Source: CAD feature listing. Evaluate the final solid. Frame: model axes, mm. A direction names the side the tool comes from. Coordinates: 2 decimals unless noted, no trailing zeros. Write each loop counter-clockwise with the first axis right and the second up, starting at its lowest first coordinate (ties: lowest second). Pieces come first, ordered by that corner, then holes. Notation, with made-up numbers: M -29,-36.75 L -11,-36.75 A6 ccw -11,-29.75 Z; hole C 73,-40 d11. An arc over 180 degrees is marked long. One line per item, written item: value. Start each with the question number.
Item 1: Ray query, L1, parallel to X at y = 0, z = 101.75; L2, parallel to Y at x = 0, z = 94.5; L3, parallel to Z at x = 5, y = 5.5. Return the intervals inside material, ascending. Write a range as from..to.
Item 2: Pin query (flat end, axial travel): P1, Ø5, axis at y = -1, z = 36, coming from the -X side (3 decimals); P2, Ø10.5, axis at y = -2.5, z = 17.5, coming from the -X side; P3, Ø5, axis at x = 20, z = 85, coming from the -Y side. Return the tip coordinate at first contact, or that it passes through.
Item 3: Cut plane A-A, the plane z = 18.5. Output: boundary loops of the cut face in (x, y), then the cut area to 3 significant figures.
Item 4: Set-up query: faces 4 (the flat face through (-7.89, -13.92, 15.91)), 5 (the flat face through (-6, -16, 91)), 6 (the conical face through (-14.35, 8.33, 22.16)), 7 (the flat face through (-16, 0, 100)). Return all of +Z, -Z, +X, -X, +Y, -Y with unobstructed straight access to the full face (end or side cutting, diameter ignored); none if empty.
Item 5: Cut plane B-B, the plane z = 81. Output: boundary loops of the cut face in (x, y).
Item 6: Mould query, pull axis Y, two halves, no side actions, for faces 1 (the conical face through (-11.986, -1.574, 38.389)), 2 (the flat face through (-17, -9, 45)), 3 (the flat face through (-7.89, 13.92, 99.62)). Classes: released by +Y, released by -Y, zero draft, split by the parting line, or undercut.
```python
from build123d import *

# Parameters (mm, degrees)
SKETCH_2_R          = 33
SKETCH_2_W          = 44
SKETCH_2_H          = 22
CUT_EXTRUDE_1_DEPTH = 6.5
SKETCH_3_R          = 33
SKETCH_3_W          = 22
SKETCH_3_H          = 44
CUT_EXTRUDE_2_DEPTH = 6.5
SKETCH_5_R          = 32
CUT_EXTRUDE_3_DEPTH = 17
SKETCH_7_R          = 32
CUT_EXTRUDE_4_DEPTH = 13


with BuildPart() as part:
    # 草图1 → 旋转1 (revolve)
    with BuildSketch(Plane(origin=(0, 0, 0), x_dir=(0, 0, -1), z_dir=(1, 0, 0))):
        Polygon((-83, 0), (-83, 10.188), (-107.188, 10.188), (-108, 11), (-108, 16), (-106.57093764, 18.475208614), (-91.6, 18.475208614), (-91, 19.075208614), (-91, 24.5), (-89, 26.5), (-52, 26.5), (-45, 22.933321854), (-45, 10.5), (-38.5, 10.5), (-38.5, 11.8), (-38.3, 12), (-32.2, 12), (-32, 11.8), (-32, 11), (-0.92, 11), (0, 10.08), (0, 0), align=None)
    revolve(axis=Axis((0, 0, 0), (0, 0, 1)))

    # 草图2 → 切除-拉伸1 (cut)
    with BuildSketch(Plane(origin=(0, 0, 32), x_dir=(-1, 0, 0), z_dir=(0, 0, -1))):
        Circle(SKETCH_2_R)
        Rectangle(SKETCH_2_W, SKETCH_2_H, mode=Mode.SUBTRACT)
    extrude(amount=-CUT_EXTRUDE_1_DEPTH, mode=Mode.SUBTRACT)

    # 草图3 → 切除-拉伸2 (cut)
    with BuildSketch(Plane(origin=(0, 0, 32), x_dir=(-1, 0, 0), z_dir=(0, 0, -1))):
        Circle(SKETCH_3_R)
        Rectangle(SKETCH_3_W, SKETCH_3_H, mode=Mode.SUBTRACT)
    extrude(amount=-CUT_EXTRUDE_2_DEPTH, mode=Mode.SUBTRACT)

    # 草图4 → 旋转2 (revolve)
    with BuildSketch(Plane(origin=(0, 0, 0), x_dir=(0, 0, -1), z_dir=(1, 0, 0))):
        with BuildLine():
            Line((-45, 19), (-45, 10.5))
            Line((-45, 10.5), (-38.5, 10.5))
            Line((-38.5, 10.5), (-38.5, 11.8))
            Line((-38.5, 11.8), (-36.726286637, 16.418867925))
            ThreePointArc((-36.726286637, 16.418867925), (-36.934089571, 18.176069017), (-38.5, 19))
            Line((-38.5, 19), (-45, 19))
        make_face()
    revolve(axis=Axis((0, 0, -50), (0, 0, 1)))

    # 草图5 → 切除-拉伸3 (cut)
    with BuildSketch(Plane.XY.offset(108)):
        Circle(SKETCH_5_R)
        Polygon((0, -18.475208614), (16, -9.237604307), (16, 9.237604307), (0, 18.475208614), (-16, 9.237604307), (-16, -9.237604307), align=None, mode=Mode.SUBTRACT)
    extrude(amount=-CUT_EXTRUDE_3_DEPTH, mode=Mode.SUBTRACT)

    # 草图6 → 旋转3 (revolve)
    with BuildSketch(Plane(origin=(0, 0, 0), x_dir=(0, 0, -1), z_dir=(1, 0, 0))):
        Polygon((-22.5, 16), (-22.5, 11), (-21.688, 10.188), (-10.312, 10.188), (-9.5, 11), (-9.5, 16), (-10.92906236, 18.475208614), (-21.07093764, 18.475208614), align=None)
    revolve(axis=Axis((0, 0, 9.5), (0, 0, 1)))

    # 草图7 → 切除-拉伸4 (cut)
    with BuildSketch(Plane(origin=(0, 0, 9.5), x_dir=(-1, 0, 0), z_dir=(0, 0, -1))):
        Circle(SKETCH_7_R)
        Polygon((0, -18.475208614), (16, -9.237604307), (16, 9.237604307), (0, 18.475208614), (-16, 9.237604307), (-16, -9.237604307), align=None, mode=Mode.SUBTRACT)
    extrude(amount=-CUT_EXTRUDE_4_DEPTH, mode=Mode.SUBTRACT)


solid = part.part
```
From the geometry:
1. L1: x = -16..-10.19, 10.19..16
1. L2: y = -18.48..-10.19, 10.19..18.48
1. L3: z = 0..83
2. P1: stops at x = -18.995
2. P2: stops at x = -16
2. P3: stops at y = -19.9
3. outline: M -16,-9.24 L 0,-18.48 L 16,-9.24 L 16,9.24 L 0,18.48 L -16,9.24 Z
3. area: 887 mm²
4. face 4: -Z, -X, -Y
4. face 5: +Z
4. face 6: -X, +Y
4. face 7: +Z, -X, +Y, -Y
5. outline: C 0,0 d53
6. face 1: undercut
6. face 2: zero draft
6. face 3: released by +Y
